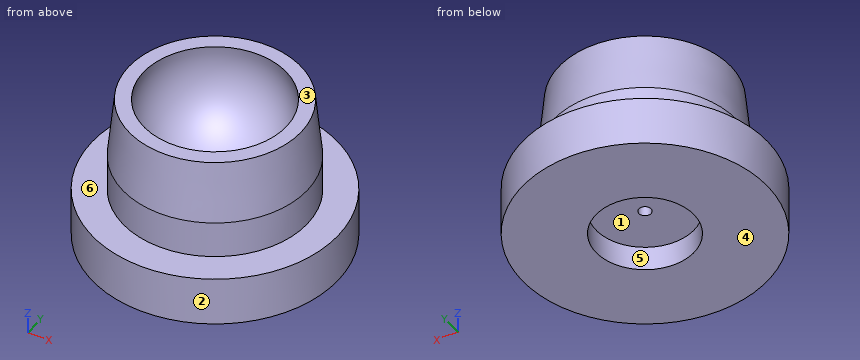
```python
from build123d import *

# Parameters (mm, degrees)
SKETCH_1_R          = 10
EXTRUDE_1_DEPTH     = 4
SKETCH_3_R          = 7
EXTRUDE_2_DEPTH     = 12
SKETCH_4_R          = 7.5
EXTRUDE_3_DEPTH     = 3
SKETCH_5_R          = 4
CUT_EXTRUDE_1_DEPTH = 2
SKETCH_6_R          = 0.5
CUT_EXTRUDE_2_DEPTH = 18.320508076
CUT_EXTRUDE_START   = -1.5
SKETCH_7_R          = 2
CUT_EXTRUDE_3_DEPTH = 16.820508076


# Read off the part's stored shape, not the designer's step: 边界1
with BuildPart() as part:
    # 草图1 → 凸台-拉伸1 (new body)
    with BuildSketch(Plane.XY):
        Circle(SKETCH_1_R)
    extrude(amount=EXTRUDE_1_DEPTH)

    # 草图3 → 凸台-拉伸2 (add)
    with BuildSketch(Plane.XY):
        Circle(SKETCH_3_R)
    extrude(amount=EXTRUDE_2_DEPTH)

    # 草图4 → 凸台-拉伸3 (add)
    with BuildSketch(Plane.XY.offset(4)):
        Circle(SKETCH_4_R)
    extrude(amount=EXTRUDE_3_DEPTH)

    # 边界1 outline → 边界1 (revolve)
    with BuildSketch(Plane.XZ):
        Polygon((7.5, 7), (7, 12), (7, 7), align=None)
    revolve(axis=Axis((0, 0, 0), (0, 0, 1)))

    # 草图5 → 切除-拉伸1 (cut)
    with BuildSketch(Plane(origin=(0, 0, 0), x_dir=(-1, 0, 0), z_dir=(0, 0, -1))):
        Circle(SKETCH_5_R)
    extrude(amount=-CUT_EXTRUDE_1_DEPTH, mode=Mode.SUBTRACT)

    # 草图6 → 切除-拉伸2 (cut, through all)
    with BuildSketch(Plane(origin=(0, 0, 2), x_dir=(-1, 0, 0), z_dir=(0, 0, -1))):
        Circle(SKETCH_6_R)
    extrude(amount=-CUT_EXTRUDE_2_DEPTH, mode=Mode.SUBTRACT)

    # 草图7 → 切除-拉伸3 (cut, through all)
    with BuildSketch(Plane(origin=(0, 0, 2), x_dir=(-1, 0, 0), z_dir=(0, 0, -1)).offset(CUT_EXTRUDE_START)):
        Circle(SKETCH_7_R)
    extrude(amount=-CUT_EXTRUDE_3_DEPTH, mode=Mode.SUBTRACT)

    # 草图8 → 切除-旋转1 (revolve, cut)
    with BuildSketch(Plane(origin=(0, 0, 0), x_dir=(0, 0, -1), z_dir=(1, 0, 0)), mode=Mode.PRIVATE) as cut_revolve_1_sk:
        with BuildLine():
            Line((-12, 0), (-12, 5.809475019))
            ThreePointArc((-12, 5.809475019), (-6.825765386, 4.74341649), (-4.5, 0))
            Line((-4.5, 0), (-12, 0))
        make_face()
    revolve(cut_revolve_1_sk.sketch.rotate(Axis((0, 0, 12), (0, 0, 1)), 286.935860908), axis=Axis((0, 0, 12), (0, 0, 1)), mode=Mode.SUBTRACT)


solid = part.part
```
Part model, mm, in its own coordinate system. Face numbers are marked on the shaded views. A direction names the side the tool comes from. Round coordinates to 2 decimals unless told otherwise and drop trailing zeros. Loops run counter-clockwise (first coordinate to the right, second up) from the corner with the lowest first, then second, coordinate; pieces in that order, holes last.
1. Drill centre lines: line 1 along Y through (x, z) = (0, 3.8); line 2 along Y through (x, z) = (0, 0.8); line 3 along X through (y, z) = (-3.5, 0.5). Where is each one in solid material? Low to high.
Solutions:
line 1: y = -10 to -2, 2 to 10
line 2: y = -10 to -4, 4 to 10
line 3: x = -9.37 to -1.94, 1.94 to 9.37
2. Slice it at C-C (z = 1.25). Give the cut face in (x, y).
Solutions:
outline: circle Ø20 at (0, 0); hole circle Ø8 at (0, 0)
3. 3-axis set-ups, long thin cutter, end or side, ignore diameter. For the marked faces 4, 5 and 6: which of +Z, -Z, +X, -X, +Y, -Y reach the whole face in a straight line?
Solutions:
face 4: -Z, +X, -X, +Y, -Y
face 5: -Z
face 6: +Z
4. Slice it at A-A (y = 0). Give the cut face in (x, z), and give its area (3 significant figures).
Solutions:
outline: (-10, 0) - (-4, 0) - (-4, 2) - (-0.5, 2) - (-0.5, 3.5) - (-2, 3.5) - (-2, 4.84) arc R6 cw to (-5.81, 12) - (-7, 12) - (-7.5, 7) - (-7.5, 4) - (-10, 4) - close; (0.5, 2) - (4, 2) - (4, 0) - (10, 0) - (10, 4) - (7.5, 4) - (7.5, 7) - (7, 12) - (5.81, 12) arc R6 cw to (2, 4.84) - (2, 3.5) - (0.5, 3.5) - close
area: 101 mm2
5. Two-plate mould, pull along X, no slides. Class the marked faces 1, 2 and 3: pulls with the +X half, pulls with the -X half, needs draft (parallel to the pull), parting line crosses it, or undercut.
Solutions:
face 1: undercut
face 2: parting line crosses it
face 3: needs draft
6. Slice it at D-D (z = 8.75). Give the cut face in (x, y) (3 decimals), and give its area (3 significant figures).
Solutions:
outline: circle Ø14.65 at (0, 0); hole circle Ø11.478 at (0, 0)
area: 65.1 mm2
7. Flat gauge pins, fed straight in: pin 1 (4 mm diameter, centred on y = 3, z = 8, fed in from +X); pin 2 (4 mm diameter, centred on x = -1, y = 1, fed in from -Z); pin 3 (4.5 mm diameter, centred on x = 0, y = 0, fed in from +Z). Where does each tip first touch, or does it go through?
Solutions:
pin 1: stops at x = 7.39
pin 2: stops at z = 2
pin 3: stops at z = 4.94
